Work out the finished part from the listing and answer in its coordinate system (mm). Face numbers are marked on the shaded views. A direction names the side the tool comes from. Coordinates: 2 decimals unless noted, no trailing zeros. Order: outer loops, then holes, each group sorted by start corner. A loop starts at its lowest first (then second) coordinate and runs counter-clockwise, first axis right, second up. Notation, with made-up numbers: M 32,-20 L 36,-20 A26 ccw 36,3 Z; hole C 55,74 d1. An arc over 180 degrees is marked long. Use a Markdown table: item, result.
from build123d import *

# Parameters (mm, degrees)
SKETCH_2_W          = 12.724713087
SKETCH_2_H          = 37.266218859
SKETCH_2_R          = 2.75
EXTRUDE_1_DEPTH     = 4
SKETCH_3_W          = 5
SKETCH_3_H          = 13
EXTRUDE_2_DEPTH     = 4
SKETCH_4_W          = 5
SKETCH_4_H          = 13
EXTRUDE_4_DEPTH     = 9
SKETCH_5_W          = 13.3
SKETCH_5_H          = 13
EXTRUDE_5_DEPTH     = 30
CUT_EXTRUDE_2_DEPTH = 78.033997806
EXTRUDE_6_DEPTH     = 13
FILLET_4_R          = 3
SKETCH_12_W         = 31
SKETCH_12_H         = 9
CUT_EXTRUDE_3_DEPTH = 79.606298904
RIB_1_REACH         = 78.775
SKETCH_13_WALL_W    = 179.357132042
SKETCH_13_WALL_H    = 5
CHAMFER_1_SIZE      = 5
FILLET_5_R          = 1
FILLET_6_R          = 2
FILLET_7_R          = 1


with BuildPart() as part:
    # 草图2 → 凸台-拉伸1 (new body)
    with BuildSketch(Plane.XY):
        with Locations((32.137643457, -0.210903357)):
            Rectangle(SKETCH_2_W, SKETCH_2_H)
        with Locations((30.5, -12.5)):
            Circle(SKETCH_2_R, mode=Mode.SUBTRACT)
        with Locations((30.5, 12.5)):
            Circle(SKETCH_2_R, mode=Mode.SUBTRACT)
    extrude(amount=EXTRUDE_1_DEPTH)

    # 草图3 → 凸台-拉伸2 (add)
    with BuildSketch(Plane(origin=(0, 230.908781145, 0), x_dir=(-1, 0, 0), z_dir=(0, 0, 1))):
        with Locations((-41, 231.119684502)):
            Rectangle(SKETCH_3_W, SKETCH_3_H)
    extrude(amount=EXTRUDE_2_DEPTH)

    # 草图4 → 凸台-拉伸4 (add)
    with BuildSketch(Plane.XY):
        with Locations((41, -0.210903358)):
            Rectangle(SKETCH_4_W, SKETCH_4_H)
    extrude(amount=-EXTRUDE_4_DEPTH)

    # 草图5 → 凸台-拉伸5 (add)
    with BuildSketch(Plane(origin=(43.5, 0, 0), x_dir=(0, 0, -1), z_dir=(1, 0, 0))):
        with Locations((2.35, -0.210903358)):
            Rectangle(SKETCH_5_W, SKETCH_5_H)
    extrude(amount=EXTRUDE_5_DEPTH)

    # 草图9 → 切除-拉伸2 (cut, through all)
    with BuildSketch(Plane.XY.offset(4.3)):
        with BuildLine():
            Line((68.5, 1.789096642), (73.5, 1.789096642))
            Line((73.5, 1.789096642), (73.5, -2.210903358))
            Line((73.5, -2.210903358), (68.5, -2.210903358))
            ThreePointArc((68.5, -2.210903358), (66.5, -0.210903358), (68.5, 1.789096642))
        make_face()
    extrude(amount=-CUT_EXTRUDE_2_DEPTH, mode=Mode.SUBTRACT)

    # 草图10 → 凸台-拉伸6 (add)
    with BuildSketch(Plane.XZ.offset(6.710903358)):
        Polygon((43.5, 11.286784974), (55.972995456, 12.130267128), (63.5, 4.3), (43.5, 4.3), align=None)
    extrude(amount=-EXTRUDE_6_DEPTH)

    # 圆角4
    fillet_4_edges = [part.edges().sort_by_distance(p)[0] for p in [
        (55.972995456, -0.210903358, 12.130267128),
    ]]
    fillet(fillet_4_edges, radius=FILLET_4_R)

    # 草图12 → 切除-拉伸3 (cut, through all)
    with BuildSketch(Plane.XZ.offset(6.710903358)):
        with Locations((58, -4.5)):
            Rectangle(SKETCH_12_W, SKETCH_12_H)
    extrude(amount=-CUT_EXTRUDE_3_DEPTH, mode=Mode.SUBTRACT)

    # 草图13 wall → 筋1 (add, up to next)
    with BuildSketch(Plane(origin=(53.519716797, -0.210903358, -4.5), x_dir=(-0.925784246104, 0, -0.378052284302), z_dir=(0.378052284302, 0, -0.925784246104)), mode=Mode.PRIVATE) as rib_1_sk1:
        Rectangle(SKETCH_13_WALL_W, SKETCH_13_WALL_H)
    rib_1_tool1 = extrude(rib_1_sk1.sketch, amount=-RIB_1_REACH, mode=Mode.PRIVATE) - part.part
    add(rib_1_tool1.solids().sort_by_distance((53.519716797, -0.210903358, -4.5))[0])

    # 倒角1
    chamfer_1_edges = [part.edges().sort_by_distance(p)[0] for p in [
        (43.5, -0.210903358, 4),
    ]]
    chamfer(chamfer_1_edges, length=CHAMFER_1_SIZE)

    # 圆角5
    fillet_5_edges = [part.edges().sort_by_distance(p)[0] for p in [
        (43.5, -0.210903358, 9),
        (43.5, -0.210903358, 11.286784974),
    ]]
    fillet(fillet_5_edges, radius=FILLET_5_R)

    # 圆角6
    fillet_6_edges = [part.edges().sort_by_distance(p)[0] for p in [
        (73.5, 1.789096642, 2.15),
        (73.5, -2.210903358, 2.15),
        (73.5, 6.289096642, 2.15),
        (73.5, -6.710903358, 2.15),
    ]]
    fillet(fillet_6_edges, radius=FILLET_6_R)

    # 圆角7
    fillet_7_edges = [part.edges().sort_by_distance(p)[0] for p in [
        (70, 1.789096642, 4.3),
        (67.5, -6.710903358, 4.3),
        (73.5, -4.460903358, 4.3),
        (73.5, 4.039096642, 4.3),
        (67.5, 6.289096642, 4.3),
        (72.914213562, -6.12511692, 4.3),
        (72.914213562, 5.703310205, 4.3),
        (72.914213562, -2.796689795, 4.3),
        (72.914213562, 2.37488308, 4.3),
        (66.5, -0.210903358, 4.3),
        (70, -2.210903358, 4.3),
    ]]
    fillet(fillet_7_edges, radius=FILLET_7_R)


solid = part.part
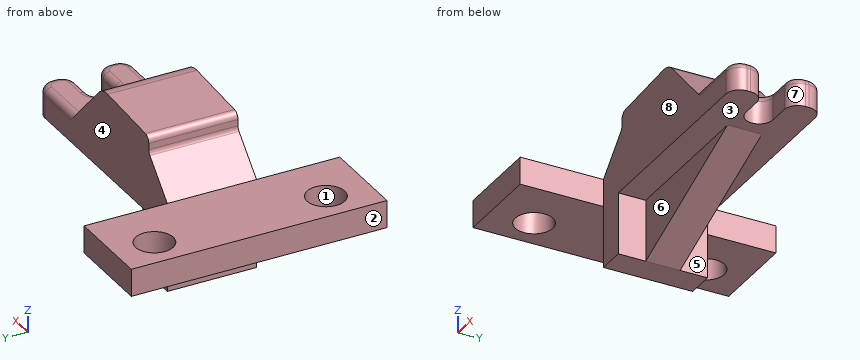
1. Section C-C on x = 30.5 is taken. Determine the outline of the cut face in (y, z), then the cut area to 3 significant figures.
Answers below:
| item | result |
|---|---|
| outline | M -18.84,0 L -15.25,0 L -15.25,4 L -18.84,4 Z; M -9.75,0 L 9.75,0 L 9.75,4 L -9.75,4 Z; M 15.25,0 L 18.42,0 L 18.42,4 L 15.25,4 Z |
| area | 105 mm² |
2. For a pull along X with two mould halves and no side action, classify the marked faces 1, 2 and 3 as +X half, -X half, draft (parallel to the pull), parting line (faces both ways), or undercut.
Answers below:
| item | result |
|---|---|
| face 1 | undercut |
| face 2 | -X half |
| face 3 | draft |
3. For the marked faces 4, 5, 6, 7 and 8, determine the directions among +Z, -Z, +X, -X, +Y, -Y from which every point of the face is accessible in a straight line to the end or side of a thin tool.
Answers below:
| item | result |
|---|---|
| face 4 | +Z, -Z, +X, +Y |
| face 5 | -Z, +X, +Y |
| face 6 | -Z, +X, -Y |
| face 7 | +Z, -Z, +X |
| face 8 | +Z, -Z, +X, -Y |
4. Section A-A on x = 70 is taken. Determine the outline of the cut face in (y, z), then the cut area to 3 significant figures.
Answers below:
| item | result |
|---|---|
| outline | M -6.71,0 L -2.21,0 L -2.21,3.3 A1 ccw -3.21,4.3 L -5.71,4.3 A1 ccw -6.71,3.3 Z; M 1.79,0 L 6.29,0 L 6.29,3.3 A1 ccw 5.29,4.3 L 2.79,4.3 A1 ccw 1.79,3.3 Z |
| area | 37.8 mm² |
5. Section D-D on z = 1 is taken. Determine the outline of the cut face in (x, y).
Answers below:
| item | result |
|---|---|
| outline | M 25.78,-18.84 L 38.5,-18.84 L 38.5,-6.71 L 71.5,-6.71 A2 ccw 73.5,-4.71 L 73.5,-4.21 A2 ccw 71.5,-2.21 L 68.5,-2.21 A2 cw 68.5,1.79 L 71.5,1.79 A2 ccw 73.5,3.79 L 73.5,4.29 A2 ccw 71.5,6.29 L 38.5,6.29 L 38.5,18.42 L 25.78,18.42 Z; hole C 30.5,-12.5 d5.5; hole C 30.5,12.5 d5.5 |
6. Flat-ended cylindrical pins translate along their axes: P1, Ø12, axis at x = 38, y = -2.5, coming from the -Z side; P2, Ø10, axis at x = 30, y = -3, coming from the -Z side; P3, Ø6.5, axis at x = 60, y = -2.5, coming from the -Z side; P4, Ø1, axis at x = 63.5, z = 2.5, coming from the -Y side. Find the tip coordinate at first contact, or state that the pin passes through.
Answers below:
| item | result |
|---|---|
| P1 | z = -9 |
| P2 | z = 0 |
| P3 | z = -3.18 |
| P4 | y = -6.71 |
7. Find the intervals of material crossed by probe 1 along Y at (x, z) = (30.5, 1.3); probe 2 along Z at (x, y) = (32.5, 7); probe 3 along X at (y, z) = (-9, 1.25), in increasing order.
Answers below:
| item | result |
|---|---|
| probe 1 | -18.84 to -15.25, -9.75 to 9.75, 15.25 to 18.42 |
| probe 2 | 0 to 4 |
| probe 3 | 25.78 to 38.5 |
8. Section B-B on y = -12.5 is taken. Determine the outline of the cut face in (x, z), then the cut area to 3 significant figures.
Answers below:
| item | result |
|---|---|
| outline | M 25.78,0 L 27.75,0 L 27.75,4 L 25.78,4 Z; M 33.25,0 L 38.5,0 L 38.5,4 L 33.25,4 Z |
| area | 28.9 mm² |
